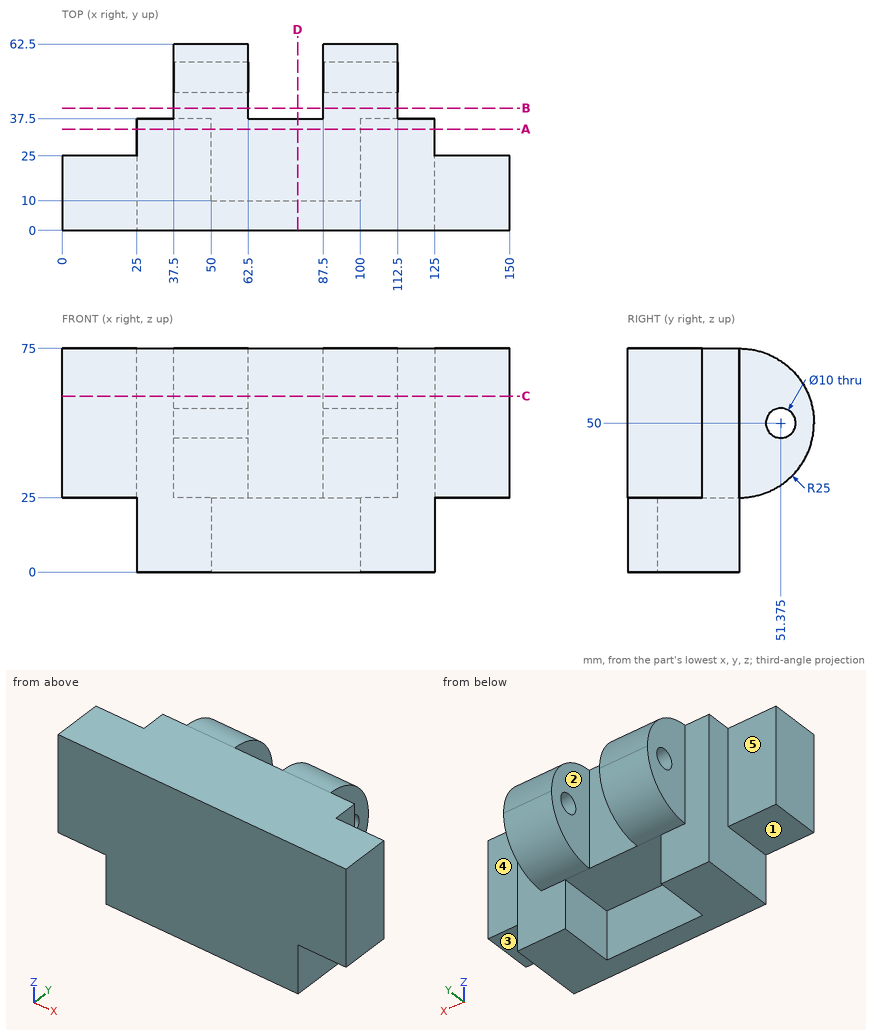
The drawing under review shows one solid part. Ordinate dimensions are in mm from its lowest x, y, z. A direction names the side the tool comes from. Round coordinates to 2 decimals unless told otherwise and drop trailing zeros. Order: outer loops, then holes, each group sorted by start corner. A loop starts at its lowest first (then second) coordinate and runs counter-clockwise, first axis right, second up. Notation, with made-up numbers: (5, 41) - (15, 41) arc R24 ccw to (15, 60) - close; hole circle Ø10 at (75, 12.5). An arc over 180 degrees is marked (long way). Return JSON: item names as keys, results as strings.
Q1. Consider section B-B on y = 41. Write out the cut boundary in (x, z), plus the area to 3 significant figures.
Computed values:
{"outline": "(37.5, 25.25) - (62.5, 25.25) - (62.5, 74.75) - (37.5, 74.75) - close; (87.5, 25.25) - (112.5, 25.25) - (112.5, 74.75) - (87.5, 74.75) - close", "area": "2,480 mm2"}
Q2. Wall thickness on L1, parallel to X at y = 43, z = 27.5; L2, parallel to X at y = 34.5, z = 7.5; L3, parallel to Y at x = 42, z = 8.5: over which ranges is each line inside the solid? List them lowest first. Write a range as [from, to].
Computed values:
{"L1": "x = [37.5, 62.5], [87.5, 112.5]", "L2": "x = [25, 50], [100, 125]", "L3": "y = [0, 37.5]"}
Q3. Consider section C-C on z = 59. Write out the cut boundary in (x, y), plus the area to 3 significant figures.
Computed values:
{"outline": "(0, 0) - (150, 0) - (150, 25) - (125, 25) - (125, 37.5) - (112.5, 37.5) - (112.5, 60.82) - (87.5, 60.82) - (87.5, 37.5) - (62.5, 37.5) - (62.5, 60.82) - (37.5, 60.82) - (37.5, 37.5) - (25, 37.5) - (25, 25) - (0, 25) - close", "area": "6,170 mm2"}
Q4. For pin 1 Ø4 at (x, z) = (128, 22) entering from -Y; pin 2 Ø7.5 at (x, z) = (139, 50.5) entering from +Y; pin 3 Ø10 at (x, z) = (73.5, 16.5) entering from +Y; pin 4 Ø7.5 at (y, z) = (29, 14.5) entering from +X, all flat-tipped, find the tip position at first contact; note any pin that passes through.
Computed values:
{"pin 1": "passes through", "pin 2": "stops at y = 25", "pin 3": "stops at y = 10", "pin 4": "stops at x = 125"}
Q5. Consider section A-A on y = 34. Write out the cut boundary in (x, z), plus the area to 3 significant figures.
Computed values:
{"outline": "(25, 0) - (50, 0) - (50, 25) - (100, 25) - (100, 0) - (125, 0) - (125, 75) - (25, 75) - close", "area": "6,250 mm2"}
Q6. Consider section D-D on x = 79. Write out the cut boundary in (y, z), plus the area to 4 significant figures.
Computed values:
{"outline": "(0, 0) - (10, 0) - (10, 25) - (37.5, 25) - (37.5, 75) - (0, 75) - close", "area": "2,125 mm2"}
Q7. Machinability: for the marked faces 1, 2, 3, 4 and 5, which of the approach directions +Z, -Z, +X, -X, +Y, -Y give a long, thin tool a straight path to every point of the face, cutting with its end or side? Answer none if there is none.
Computed values:
{"face 1": "-Z, -X, +Y, -Y", "face 2": "+Z, -Z, +Y", "face 3": "-Z, +X, +Y, -Y", "face 4": "+Z, -Z, +X, +Y", "face 5": "+Z, -Z, -X, +Y"}
